Input: part model. Units: mm. Frame: model coordinates. A direction names the side the tool comes from. Round coordinates to 2 decimals unless told otherwise and drop trailing zeros. Loops run counter-clockwise (first coordinate to the right, second up) from the corner with the lowest first, then second, coordinate; pieces in that order, holes last.
1) Ray query, line 1 along Y through (x, z) = (23.25, -12.7) (3 decimals); line 2 along Z through (x, y) = (-22, 57.5); line 3 along X through (y, z) = (58.5, 0). Return the intervals inside material, ascending.
2) Section C-C, the plane z = 12.7. State how many separate pieces and enclosed holes the cut face has, and give its area (3 significant figures).
3) First-contact query: pin 1 (3 mm diameter, centred on x = 22, z = -24.71, fed in from +Y); pin 2 (4.5 mm diameter, centred on x = -23.34, z = 23.57, fed in from -Y); pin 3 (5 mm diameter, centred on y = 15.875, z = 12.7, fed in from +X). Flat tips, straight axial feed; report the tip coordinate or a pass-through.
4) Section D-D, the plane y = 17.5. Return loops of the section in (x, z).
5) Access query for faces 4 (the face through (13, 69.85, 13)), 5 (the face through (23.46, 56.97, 24.34)), 6 (the face through (-20.9, 12.9, 24.1)), 7 (the face through (-22, 35, -9.525)), 8 (the face through (20.65, 53.149, -15.323)). Directions: +Z, -Z, +X, -X, +Y, -Y. A direction counts if a zero-diameter tool reaches every point of the face in a straight line with its end or side. Return the directions, or none.
6) Draft query along X for faces 1 (the face through (-26.22, 35.41, -26.32)), 2 (the face through (0, 34, -28.13)), 3 (the face through (-22.39, 12.88, -25.88)). Return one class per face: pulls with the +X half, pulls with the -X half, needs draft (parallel to the pull), parting line crosses it, or undercut.
Autodesk Inventor part; units mm, degrees
ref_plane "YZ Plane" through (0, 0, 0) normal (1, 0, 0) x (0, 1, 0)
ref_plane "XZ Plane" through (0, 0, 0) normal (0, 1, 0) x (-1, 0, 0)
ref_plane "XY Plane" through (0, 0, 0) normal (0, 0, 1) x (1, 0, 0)
sketch "Sketch1" plane through (0, 0, 0) normal (0, 1, 0) x (-1, 0, 0)
  line L0 (28.1305, 28.1305) -> (-28.1305, 28.1305)
  line L1 (-28.1305, 28.1305) -> (-28.1305, -28.1305)
  line L2 (-28.1305, -28.1305) -> (28.1305, -28.1305)
  line L3 (28.1305, -28.1305) -> (28.1305, 28.1305)
  line L4 (28.1305, 28.1305) -> (-28.1305, -28.1305) construction
  line L5 (-28.1305, 28.1305) -> (28.1305, -28.1305) construction
  point P0 (0, 0)
  dimension "d0" = 56.261
  dimension "d1" = 56.261
extrude "Extrusion1" add sketch "Sketch1" along normal blind 69.85
sketch "Sketch2" plane through (0, 69.85, 0) normal (0, 1, 0) x (1, 0, 0)
  circle A0 centre (0, 0) radius 18
  point P0 (-22, 24.7091)
  point P1 (22, 24.7091)
  point P2 (24.0589, -22.4333)
  point P3 (-22, -19.2909)
  dimension "d4" = 44
  dimension "d5" = 44
  dimension "d6" = 22
  dimension "d7" = 36
hole "Hole1" at (-22, 69.85, -24.7091) at (22, 69.85, -24.7091) at (24.0589, 69.85, 22.4333) at (-22, 69.85, 19.2909) direction (0, -1, 0) diameter 4 depth 25.4 tip angle 118
sketch "Sketch3" plane through (0, 69.85, 0) normal (0, 1, 0) x (1, 0, 0)
  circle A0 centre (0, 0) radius 18
  dimension "d15" = 36
extrude "Extrusion2" cut sketch "Sketch3" against normal blind 254
sketch "Sketch4" plane through (0, 0, 0) normal (0, -1, 0) x (1, 0, 0)
  circle A0 centre (0, 0) radius 18
  point P0 (-23.3446, 23.5712)
  point P1 (23.7978, 23.5712)
  point P2 (23.7978, -23.5712)
  point P3 (-23.3446, -23.5712)
  dimension "d18" = 47.1424
  dimension "d19" = 47.1424
  dimension "d20" = 23.5712
hole "Hole2" at (-23.3446, 0, 23.5712) at (23.7978, 0, 23.5712) at (23.7978, 0, -23.5712) at (-23.3446, 0, -23.5712) direction (0, 1, 0) diameter 5 depth 25.4 tip angle 118
sketch "Sketch5" plane through (0, 0, 0) normal (0, -1, 0) x (1, 0, 0)
  circle A0 centre (0, 0) radius 18
  circle A1 centre (0, 0) radius 19.0754
  dimension "d28" = 38.1508
extrude "Extrusion3" cut sketch "Sketch5" against normal blind 34.925
fillet "Fillet1" radius 6.35 1 edges at (28.1305, 34.925, 28.1305)
fillet "Fillet2" radius 6.35 1 edges at (-28.1305, 34.925, 28.1305)
fillet "Fillet3" radius 6.35 1 edges at (28.1305, 34.925, -28.1305)
fillet "Fillet4" radius 6.35 1 edges at (-28.1305, 34.925, -28.1305)
sketch "Sketch6" plane through (-28.1305, 0, 21.7805) normal (-1, 0, 0) x (0, 0, 1)
  line L0 (-49.911, 0) -> (0, 0)
  line L1 (0, 69.85) -> (0, 0)
  line L2 (-31.3055, 25.4) -> (-12.2555, 25.4) construction
  line L3 (-12.2555, 25.4) -> (-12.2555, 44.45)
  line L4 (-12.2555, 44.45) -> (-31.3055, 44.45) construction
  line L5 (-31.3055, 44.45) -> (-31.3055, 25.4)
  line L6 (-31.3055, 25.4) -> (-12.2555, 44.45) construction
  line L7 (-12.2555, 25.4) -> (-31.3055, 44.45) construction
  arc A0 (-12.2555, 44.45) -> (-31.3055, 44.45) centre (-21.7805, 44.45) ccw
  arc A1 (-31.3055, 25.4) -> (-12.2555, 25.4) centre (-21.7805, 25.4) ccw
  point P0 (-43.561, 0)
  point P1 (-21.7805, 0)
  point P2 (-21.7805, 34.925)
  point P3 (-21.7805, 34.925)
  point P4 (-21.7805, 0)
  point P5 (0, 34.925)
  point P6 (-21.7805, 53.975)
  point P7 (-21.7805, 15.875)
  dimension "d35" = 19.05
  dimension "d36" = 19.05
extrude "Extrusion4" cut sketch "Sketch6" against normal blind 25.4
sketch "Sketch7" plane through (28.1305, 0, 21.7805) normal (1, 0, 0) x (0, 0, -1)
  line L0 (0, 0) -> (0, 69.85)
  line L1 (0, 0) -> (49.911, 0)
  line L2 (9.0805, 15.875) -> (34.4805, 15.875) construction
  line L3 (34.4805, 15.875) -> (34.4805, 53.975) construction
  line L4 (34.4805, 53.975) -> (9.0805, 53.975) construction
  line L5 (9.0805, 53.975) -> (9.0805, 15.875) construction
  line L6 (9.0805, 15.875) -> (34.4805, 53.975) construction
  line L7 (34.4805, 15.875) -> (9.0805, 53.975) construction
  line L8 (0, 69.85) -> (49.911, 69.85)
  point P0 (43.561, 0)
  point P1 (21.7805, 0)
  point P2 (21.7805, 34.925)
  point P3 (21.7805, 0)
  point P4 (0, 34.925)
  point P5 (43.561, 69.85)
  dimension "d39" = 25.4
  dimension "d40" = 38.1
  dimension "d48" = 15.875
hole "Hole3" at (28.1305, 53.975, 12.7) at (28.1305, 53.975, -12.7) at (28.1305, 15.875, -12.7) at (28.1305, 15.875, 12.7) direction (-1, 0, 0) diameter 5.5 depth 25.4 tip angle 118
properties part number "nema23_motor_mount"
Final values:
1. line 1: y = 0 to 13.125, 18.625 to 51.225, 56.725 to 69.85
1. line 2: z = -28.13 to -26.71, -22.71 to 17.29, 21.29 to 28.13
1. line 3: x = -28.13 to -18, 18 to 28.13
2. separate pieces: 4
2. enclosed holes: 0
2. area: 1,880 mm2
3. pin 1: stops at y = 44.15
3. pin 2: stops at y = 25.55
3. pin 3: stops at x = -11.53
4. outline: (-28.13, -21.78) arc R6.35 ccw to (-21.78, -28.13) - (21.78, -28.13) arc R6.35 ccw to (28.13, -21.78) - (28.13, -14.92) - (11.89, -14.92) arc R19.08 cw to (-18.32, -5.32) - (-28.13, -5.32) - close; (-28.13, 5.32) - (-18.32, 5.32) arc R19.08 cw to (11.89, 14.92) - (28.13, 14.92) - (28.13, 21.78) arc R6.35 ccw to (21.78, 28.13) - (-21.78, 28.13) arc R6.35 ccw to (-28.13, 21.78) - close; (15.94, -10.48) - (28.13, -10.48) - (28.13, 10.48) - (15.94, 10.48) arc R19.08 cw to start; hole circle Ø5 at (-23.34, -23.57); hole circle Ø5 at (-23.34, 23.57); hole circle Ø5 at (23.8, -23.57); hole circle Ø5 at (23.8, 23.57)
5. face 4: +Z, -Z, +X, -X, +Y
5. face 5: +Y
5. face 6: -Y
5. face 7: -X
5. face 8: +X
6. face 1: pulls with the -X half
6. face 2: needs draft
6. face 3: undercut
